Autodesk Inventor part; units mm, degrees
ref_plane "YZ Plane" through (0, 0, 0) normal (1, 0, 0) x (0, 1, 0)
ref_plane "XZ Plane" through (0, 0, 0) normal (0, 1, 0) x (-1, 0, 0)
ref_plane "XY Plane" through (0, 0, 0) normal (0, 0, 1) x (1, 0, 0)
sketch "Sketch1" plane through (0, 0, 0) normal (0, 1, 0) x (-1, 0, 0)
  line L0 (6, 8) -> (-6, 8)
  line L1 (-8, 6) -> (-8, -6)
  line L2 (-6, -8) -> (6, -8)
  line L3 (8, -6) -> (8, 6)
  arc A0 (8, 6) -> (6, 8) centre (6, 6) ccw
  arc A1 (-6, 8) -> (-8, 6) centre (-6, 6) ccw
  arc A2 (-8, -6) -> (-6, -8) centre (-6, -6) ccw
  arc A3 (6, -8) -> (8, -6) centre (6, -6) ccw
  point P0 (0, 0)
  point P1 (8, 8)
  point P2 (-8, 8)
  point P3 (8, -8)
  dimension "d0" = 16
  dimension "d1" = 16
  dimension "d2" = 8
  dimension "d3" = 8
  dimension "d4" = 2
extrude "Extrusion1" add sketch "Sketch1" along normal blind 43
sketch "Sketch2" plane through (0, 0, 0) normal (0, -1, 0) x (1, 0, 0)
  point P0 (0, 0)
hole "Hole1" at (0, 0, 0) direction (0, 1, 0) diameter 6.756 end through all
sketch "Sketch3" plane through (0, 43, 0) normal (0, 1, 0) x (1, 0, 0)
  line L0 (-6, 1.5) -> (-6, -1.5) construction
  line L1 (-6.65, 1.5) -> (-6.65, -1.5)
  line L2 (-5.35, -1.5) -> (-5.35, 1.5)
  arc A0 (-5.35, 1.5) -> (-6.65, 1.5) centre (-6, 1.5) ccw
  arc A1 (-6.65, -1.5) -> (-5.35, -1.5) centre (-6, -1.5) ccw
  line L3 (6, 1.5) -> (6, -1.5) construction
  line L4 (5.35, 1.5) -> (5.35, -1.5)
  line L5 (6.65, -1.5) -> (6.65, 1.5)
  arc A2 (6.65, 1.5) -> (5.35, 1.5) centre (6, 1.5) ccw
  arc A3 (5.35, -1.5) -> (6.65, -1.5) centre (6, -1.5) ccw
  line L6 (-6, 0) -> (6, 0) construction
  line L7 (6, 8) -> (-6, 8)
  point P0 (0, 0)
  dimension "d25" = 0.65
  dimension "d26" = 0.65
  dimension "d27" = 3
  dimension "d29" = 0
  dimension "d30" = 12
  dimension "d31" = 6
  dimension "d32" = 3
extrude "Extrusion3" add sketch "Sketch3" along normal blind 1.5
sketch "Sketch4" plane through (0, 0, 0) normal (0, -1, 0) x (1, 0, 0)
  line L0 (-6, 1.5) -> (-6, -1.5) construction
  line L1 (-6.65, 1.5) -> (-6.65, -1.5)
  line L2 (-5.35, -1.5) -> (-5.35, 1.5)
  arc A0 (-5.35, 1.5) -> (-6.65, 1.5) centre (-6, 1.5) ccw
  arc A1 (-6.65, -1.5) -> (-5.35, -1.5) centre (-6, -1.5) ccw
  line L3 (6, 1.5) -> (6, -1.5) construction
  line L4 (5.35, 1.5) -> (5.35, -1.5)
  line L5 (6.65, -1.5) -> (6.65, 1.5)
  arc A2 (6.65, 1.5) -> (5.35, 1.5) centre (6, 1.5) ccw
  arc A3 (5.35, -1.5) -> (6.65, -1.5) centre (6, -1.5) ccw
  line L6 (-6, 0) -> (6, 0) construction
  point P0 (0, 0)
  point P1 (0, 0)
  dimension "d35" = 0.65
  dimension "d36" = 0.65
  dimension "d37" = 3
  dimension "d38" = 0
  dimension "d39" = 12
  dimension "d40" = 6
  dimension "d41" = 3
extrude "Extrusion4" add sketch "Sketch4" along normal blind 1.5
equation "\"d26\" = d25"
equation "\"d27\" = d32"
equation "\"d36\" = d35"
equation "\"d37\" = d41"
properties part number "Camera Mount 43mm_all"
The listing builds one solid part. Answer for the finished solid, in the listing's coordinates (mm). A direction names the side the tool comes from. Round coordinates to 2 decimals unless told otherwise and drop trailing zeros. Loops run counter-clockwise (first coordinate to the right, second up) from the corner with the lowest first, then second, coordinate; pieces in that order, holes last.
Q1. Find the intervals of material crossed by line 1 (Z direction, x = 0, y = 12.5); line 2 (Y direction, x = -6.75, z = 3.5), in increasing order.
Q2. Section B-B, the plane y = 8 is taken. Determine the outline of the cut face in (x, z), then the cut area to 3 significant figures.
Q3. Which of the six approach directions +Z, -Z, +X, -X, +Y, -Y give full straight-line access (tool end or side, diameter ignored) to faces 1 (the face through (5.99, -0.74, 2.15)), 2 (the face through (-6.65, 44, 0)), 3 (the face through (-5.99, -0.74, -2.15)), 4 (the face through (6.01, 43.74, 2.15))?
Q4. Section A-A, the plane x = 0 is taken. Determine the outline of the cut face in (y, z).
Q5. For a pull along X with two mould halves and no side action, classify faces 5 (the face through (6, 44.5, 0)), 6 (the face through (6.01, -0.74, -2.15)), 7 (the face through (-5.99, 43.74, 2.15)), 8 (the face through (-6.65, -1, 0)) as released by +X, released by -X, zero draft, split by the parting line, or undercut.
Q6. Section C-C, the plane z = -0.25 is taken. Determine the outline of the cut face in (x, y), then the cut area to 3 significant figures.
Q7. Given pin 1 Ø0.8 at (y, z) = (-0.5, 0.5) entering from -X; pin 2 Ø0.8 at (y, z) = (-1, 0) entering from +X; pin 3 Ø5 at (x, z) = (-1.5, 3.5) entering from +Y; pin 4 Ø5.5 at (x, z) = (0, 0) entering from +Y, each flat-ended and moving along its own axis, determine where each tip first touches the part or whether it passes through.
Q8. Section D-D, the plane x = 2.25 is taken. Determine the outline of the cut face in (y, z), then the cut area to 3 significant figures.
Completed:
1. line 1: z = -8 to -3.38, 3.38 to 8
1. line 2: y = 0 to 43
2. outline: (-8, -6) arc R2 ccw to (-6, -8) - (6, -8) arc R2 ccw to (8, -6) - (8, 6) arc R2 ccw to (6, 8) - (-6, 8) arc R2 ccw to (-8, 6) - close; hole circle Ø6.76 at (0, 0)
2. area: 217 mm2
3. face 1: +Z, -Y
3. face 2: +Z, -Z, -X, +Y
3. face 3: -Z, -Y
3. face 4: +Z, +Y
4. outline: (0, -8) - (43, -8) - (43, -3.38) - (0, -3.38) - close; (0, 3.38) - (43, 3.38) - (43, 8) - (0, 8) - close
5. face 5: zero draft
5. face 6: undercut
5. face 7: undercut
5. face 8: released by -X
6. outline: (-8, 0) - (-6.65, 0) - (-6.65, -1.5) - (-5.35, -1.5) - (-5.35, 0) - (-3.37, 0) - (-3.37, 43) - (-5.35, 43) - (-5.35, 44.5) - (-6.65, 44.5) - (-6.65, 43) - (-8, 43) - close; (3.37, 0) - (5.35, 0) - (5.35, -1.5) - (6.65, -1.5) - (6.65, 0) - (8, 0) - (8, 43) - (6.65, 43) - (6.65, 44.5) - (5.35, 44.5) - (5.35, 43) - (3.37, 43) - close
6. area: 406 mm2
7. pin 1: stops at x = -6.65
7. pin 2: stops at x = 6.65
7. pin 3: stops at y = 43
7. pin 4: passes through
8. outline: (0, -8) - (43, -8) - (43, -2.52) - (0, -2.52) - close; (0, 2.52) - (43, 2.52) - (43, 8) - (0, 8) - close
8. area: 471 mm2
